from build123d import *

# Parameters (mm, degrees)
F0_W     = 38.1
F0_H     = 38.1
F1_DEPTH = 1.27
F3_DEPTH = 25.4
F4_R     = 1.5875
F4_R_2   = 2.54
F5_DEPTH = 25.4


with BuildPart() as f1:
    # F0 (on Top) → F1 (new body)
    with BuildSketch(Plane.XY):
        Rectangle(F0_W, F0_H)
    extrude(amount=F1_DEPTH)

    # F2 (on Top) → F3 (cut)
    with BuildSketch(Plane.XY):
        with BuildLine():
            ThreePointArc((-0.518475, 6.200063), (-1.065611, 7.141481), (-2.14087, 7.313076))
            ThreePointArc((-2.14087, 7.313076), (-6.590117, 3.82554), (-7.412157, -1.767578))
            ThreePointArc((-7.412157, -1.767578), (-6.729914, -2.616206), (-5.641081, -2.624462))
            ThreePointArc((-5.641081, -2.624462), (-5.033573, -2.026098), (-4.941438, -1.178385))
            ThreePointArc((-4.941438, -1.178385), (-4.393411, 2.55036), (-1.427246, 4.875384))
            ThreePointArc((-1.427246, 4.875384), (-0.736807, 5.375783), (-0.518475, 6.200063))
        make_face()
        with BuildLine():
            ThreePointArc((5.641081, -2.624462), (6.729914, -2.616206), (7.412157, -1.767578))
            ThreePointArc((7.412157, -1.767578), (6.590117, 3.82554), (2.14087, 7.313076))
            ThreePointArc((2.14087, 7.313076), (1.065611, 7.141481), (0.518475, 6.200063))
            ThreePointArc((0.518475, 6.200063), (0.736807, 5.375783), (1.427246, 4.875384))
            ThreePointArc((1.427246, 4.875384), (4.393411, 2.55036), (4.941438, -1.178385))
            ThreePointArc((4.941438, -1.178385), (5.033573, -2.026098), (5.641081, -2.624462))
        make_face()
        with BuildLine():
            ThreePointArc((-5.126844, -3.524921), (-5.673013, -4.4669), (-5.288787, -5.485721))
            ThreePointArc((-5.288787, -5.485721), (0, -7.62), (5.288787, -5.485721))
            ThreePointArc((5.288787, -5.485721), (5.673013, -4.4669), (5.126844, -3.524921))
            ThreePointArc((5.126844, -3.524921), (4.302789, -3.305743), (3.525858, -3.657147))
            ThreePointArc((3.525858, -3.657147), (0, -5.08), (-3.525858, -3.657147))
            ThreePointArc((-3.525858, -3.657147), (-4.302789, -3.305743), (-5.126844, -3.524921))
        make_face()
    extrude(amount=F3_DEPTH, mode=Mode.SUBTRACT)

    # F4 (on Top) → F5 (cut)
    with BuildSketch(Plane.XY):
        with Locations((13.97, 13.97)):
            Circle(F4_R)
        with Locations((13.97, -13.97)):
            Circle(F4_R)
        with Locations((-13.97, -13.97)):
            Circle(F4_R)
        with Locations((-13.97, 13.97)):
            Circle(F4_R)
        Circle(F4_R_2)
    extrude(amount=F5_DEPTH, mode=Mode.SUBTRACT)


solid = f1.part
Model file for the job. Use its own axes, mm. A direction names the side the tool comes from. Round coordinates to 2 decimals unless told otherwise and drop trailing zeros. Loops run counter-clockwise (first coordinate to the right, second up) from the corner with the lowest first, then second, coordinate; pieces in that order, holes last. Notation, with made-up numbers: M -29,-30.5 L 3,-30.5 A20 ccw 3,-6.5 Z; hole C -40,52 d1. An arc over 180 degrees is marked long. One line per question, with ' | ' between items.
1) Mould opens along Y. For faces 3 (the flat face through (4, 0, 0)), 4 (the flat face through (0, -19.05, 1)), 5 (the cylindrical face through (-14.31, 12.42, 0.63)), 6 (the cylindrical face through (-4.42, 2.5, 0.63)) say: +Y half, -Y half, draft (parallel to the pull), parting line (faces both ways), or undercut.
Solved:
face 3: draft | face 4: -Y half | face 5: undercut | face 6: undercut
2) Band-saw the part on A-A (x = 13.97). Give the cut face in (y, z), then the cut area to 3 significant figures.
Solved:
outline: M -19.05,0 L -15.56,0 L -15.56,1.27 L -19.05,1.27 Z; M -12.38,0 L 12.38,0 L 12.38,1.27 L -12.38,1.27 Z; M 15.56,0 L 19.05,0 L 19.05,1.27 L 15.56,1.27 Z | area: 40.3 mm²
3) Band-saw the part on D-D (z = 0.8). Give the number of separate pieces and of enclosed holes in the cut face, then the cut area to 3 significant figures.
Solved:
separate pieces: 1 | enclosed holes: 8 | area: 1,310 mm²
4) Drill centre lines: line 1 along X through (y, z) = (0, 0.7); line 2 along X through (y, z) = (13.97, 0.9). Where is each one in solid material? Low to high.
Solved:
line 1: x = -19.05 to -7.62, -5.08 to -2.54, 2.54 to 5.08, 7.62 to 19.05 | line 2: x = -19.05 to -15.56, -12.38 to 12.38, 15.56 to 19.05
5) 3-axis set-ups, long thin cutter, end or side, ignore diameter. For faces 1 (the cylindrical face through (0.05, -5.08, 0.63)), 2 (the flat face through (4, 0, 1.27)): which of +Z, -Z, +X, -X, +Y, -Y reach the whole face in a straight line?
Solved:
face 1: +Z, -Z | face 2: +Z, +X, -X, +Y, -Y
6) Band-saw the part on C-C (y = 0). Give the cut face in (x, z).
Solved:
outline: M -19.05,0 L -7.62,0 L -7.62,1.27 L -19.05,1.27 Z; M -5.08,0 L -2.54,0 L -2.54,1.27 L -5.08,1.27 Z; M 2.54,0 L 5.08,0 L 5.08,1.27 L 2.54,1.27 Z; M 7.62,0 L 19.05,0 L 19.05,1.27 L 7.62,1.27 Z
